Model file for the job. Use its own axes, mm. Face numbers are marked on the shaded views. Coordinates: 2 decimals unless noted, no trailing zeros. Write each loop counter-clockwise with the first axis right and the second up, starting at its lowest first coordinate (ties: lowest second). Pieces come first, ordered by that corner, then holes. Notation, with made-up numbers: (32.5, 51.25) - (72.5, 51.25) arc R16 ccw to (72.5, 68.25) - close; hole circle Ø6 at (-29.75, 69.5). An arc over 180 degrees is marked (long way). Put each result on its own line as item: value. Start each with the question number.
1. Drill centre lines: L1, parallel to Y at x = 4.75, z = -1; L2, parallel to X at y = 47.5, z = 1.5. Where is each one in solid material? Low to high. Write a range as from..to.
2. Saw through at C-C, the plane z = 2.75. Write the cut outline in (x, y).
3. Saw through at A-A, the plane y = 27.5. Write the cut outline in (x, z), plus the area to 3 significant figures.
4. Saw through at B-B, the plane x = -2.25. Write the cut outline in (y, z).
5. Pull direction Z, two halves, no side cores. Call the marked faces 1 and 2: released by +Z, released by -Z, zero draft, split by the parting line, or undercut.
6. Drop flat-ended pins along their axis: P1, Ø0.5, axis at x = 4, y = 0.5, coming from the -Z side; P2, Ø1.5, axis at y = 62.5, z = 4, coming from the +X side; P3, Ø5, axis at y = 24.5, z = 3.5, coming from the -X side. Give the stop position or say it passes through.
```python
from build123d import *

# Parameters (mm, degrees)
CROQUIS1_R              = 4
SALIENTE_EXTRUIR1_DEPTH = 85
SALIENTE_EXTRUIR2_DEPTH = 2
REDONDEO1_R             = 1
MATRIZC1_COUNT          = 4
REDONDEO1_OF_MATRIZC1_R = 1


with BuildPart() as part:
    # Croquis1 → Saliente-Extruir1 (new body)
    with BuildSketch(Plane(origin=(0, 0, 0), x_dir=(1, 0, 0), z_dir=(0, 1, 0))):
        with Locations(Location((0, 0, 0), (0, 0, 270))):
            Circle(CROQUIS1_R)
    extrude(amount=SALIENTE_EXTRUIR1_DEPTH)

    # Croquis2 → Saliente-Extruir2 (add)
    with BuildSketch(Plane.XZ):
        with BuildLine():
            Line((-1.5, 5.208099244), (1.5, 5.208099244))
            Line((1.5, 5.208099244), (1.5, 3.708099244))
            ThreePointArc((1.5, 3.708099244), (0, 4), (-1.5, 3.708099244))
            Line((-1.5, 3.708099244), (-1.5, 5.208099244))
        make_face()
    saliente_extruir2 = extrude(amount=-SALIENTE_EXTRUIR2_DEPTH)

    # Redondeo1
    redondeo1_edges = [part.edges().sort_by_distance(p)[0] for p in [
        (-1.5, 1, 5.208099244),
        (1.5, 1, 5.208099244),
    ]]
    fillet(redondeo1_edges, radius=REDONDEO1_R)

    # MatrizC1: Saliente-Extruir2 ×4 about axis
    matrizc1_axis = Axis((0, 0, 0), (0, 1, 0))
    for i in range(1, MATRIZC1_COUNT):
        add(saliente_extruir2.rotate(matrizc1_axis, i * 360 / MATRIZC1_COUNT))

    # Redondeo1 of MatrizC1
    redondeo1_of_matrizc1_edges = [part.edges().sort_by_distance(p)[0] for p in [
        (5.208099244, 1, 1.5),
        (5.208099244, 1, -1.5),
        (1.5, 1, -5.208099244),
        (-1.5, 1, -5.208099244),
        (-5.208099244, 1, -1.5),
        (-5.208099244, 1, 1.5),
    ]]
    fillet(redondeo1_of_matrizc1_edges, radius=REDONDEO1_OF_MATRIZC1_R)


solid = part.part
```
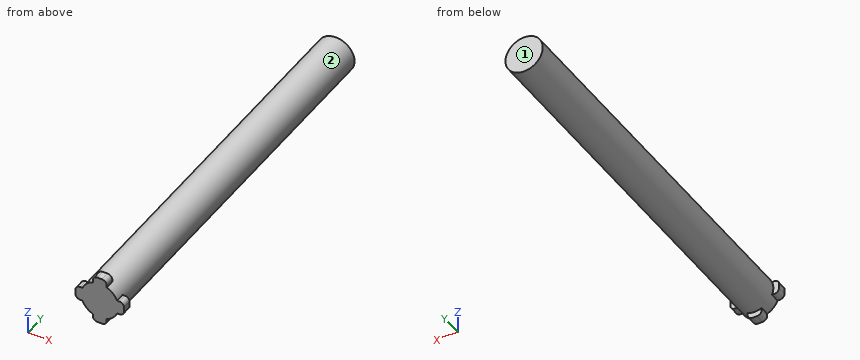
Final values:
1. L1: y = 0..2
1. L2: x = -3.71..3.71
2. outline: (-2.9, 0) - (2.9, 0) - (2.9, 85) - (-2.9, 85) - close
3. outline: circle Ø8 at (0, 0)
3. area: 50.3 mm²
4. outline: (0, -3.31) - (85, -3.31) - (85, 3.31) - (0, 3.31) - close
5. face 1: zero draft
5. face 2: split by the parting line
6. P1: stops at z = -1.5
6. P2: stops at x = 2.33
6. P3: stops at x = -3.87
